CAD build for the part. Positions are in the model's coordinates, mm. Face numbers are marked on the shaded views. A direction names the side the tool comes from. Round coordinates to 2 decimals unless told otherwise and drop trailing zeros. Order: outer loops, then holes, each group sorted by start corner. A loop starts at its lowest first (then second) coordinate and runs counter-clockwise, first axis right, second up. Notation, with made-up numbers: (65, -25.75) -> (76, -25.75) arc R13 cw to (76, -9.75) -> close; hole circle Ø4 at (77, 28). An arc over 180 degrees is marked (long way). Return JSON: item names as keys, results as strings. Group by question number.
Q1. Cut at C-C (z = -7.5). Write the cut outline in (x, y), then the cut area to 3 significant figures.
Q2. Cut at B-B (y = 0.35). Write the cut outline in (x, z), then the cut area to 3 significant figures.
Q3. Cut at D-D (x = 6.5). Write the cut outline in (y, z), then the cut area to 3 significant figures.
Q4. Mould opens along X. For the marked faces 3, 4, 5 and 6 say: +X half, -X half, draft (parallel to the pull), parting line (faces both ways), or undercut.
Q5. Which spindle directions (+Z, -Z, +X, -X, +Y, -Y) get a long thin tool onto all of the face, cutting with end or side? Do the marked faces 1 and 2. Say none if no direction does.
Q6. Cut at A-A (x = 5). Write the cut outline in (y, z), then the cut area to 3 significant figures.
Q7. Probe line 1 along X through (y, z) = (-0.2, -7.5); line 2 along X through (y, z) = (0.95, -7.5); line 3 along Z through (x, y) = (5, 0.7). List the from-to ranges inside material, lowest first.
from build123d import *

# Parameters (mm, degrees)
SKETCH1_W             = 10
SKETCH1_H             = 15
BOSS_EXTRUDE1_DEPTH   = 1.6
FILLET1_R             = 1.5
SKETCH2_R             = 3.45
BOSS_EXTRUDE2_DEPTH   = 1.4
M3X0_5_TAPPED_HOLE1_D = 2.5


with BuildPart() as part:
    # Sketch1 → Boss-Extrude1 (new body)
    with BuildSketch(Plane(origin=(0, 0, 0), x_dir=(1, 0, 0), z_dir=(0, 1, 0))):
        with Locations((5, 7.5)):
            Rectangle(SKETCH1_W, SKETCH1_H)
    extrude(amount=BOSS_EXTRUDE1_DEPTH)

    # Fillet1
    fillet1_edges = [part.edges().sort_by_distance(p)[0] for p in [
        (0, 0.8, -15),
        (10, 0.8, -15),
        (10, 0.8, 0),
        (0, 0.8, 0),
    ]]
    fillet(fillet1_edges, radius=FILLET1_R)

    # Sketch2 → Boss-Extrude2 (add)
    with BuildSketch(Plane.XZ):
        with Locations(Location((5, -7.5, 0), (0, 0, 270))):
            Circle(SKETCH2_R)
    extrude(amount=BOSS_EXTRUDE2_DEPTH)

    # M3x0.5 Tapped Hole1 (through all)
    with Locations(Plane(origin=(0, 1.6, 0), x_dir=(1, 0, 0), z_dir=(0, 1, 0))):
        with Locations((5, 7.5)):
            Hole(M3X0_5_TAPPED_HOLE1_D / 2)


solid = part.part
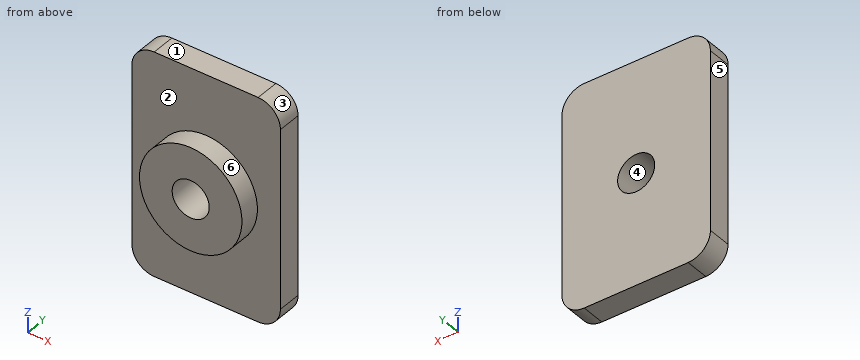
Solution:
{
 "1": {"outline": "(0, 0) -> (1.55, 0) -> (1.55, -1.4) -> (3.75, -1.4) -> (3.75, 1.6) -> (0, 1.6) -> close; (6.25, -1.4) -> (8.45, -1.4) -> (8.45, 0) -> (10, 0) -> (10, 1.6) -> (6.25, 1.6) -> close", "area": "18.2 mm²"},
 "2": {"outline": "(0, -13.5) arc R1.5 ccw to (1.5, -15) -> (8.5, -15) arc R1.5 ccw to (10, -13.5) -> (10, -1.5) arc R1.5 ccw to (8.5, 0) -> (1.5, 0) arc R1.5 ccw to (0, -1.5) -> close; hole circle Ø2.5 at (5, -7.5)", "area": "143 mm²"},
 "3": {"outline": "(-1.4, -10.61) -> (0, -10.61) -> (0, -15) -> (1.6, -15) -> (1.6, 0) -> (0, 0) -> (0, -4.39) -> (-1.4, -4.39) -> close", "area": "32.7 mm²"},
 "4": {"face 3": "+X half", "face 4": "undercut", "face 5": "-X half", "face 6": "parting line"},
 "5": {"face 1": "+Z, +X, -X, +Y, -Y", "face 2": "-Y"},
 "6": {"outline": "(-1.4, -10.95) -> (0, -10.95) -> (0, -15) -> (1.6, -15) -> (1.6, -8.75) -> (-1.4, -8.75) -> close; (-1.4, -6.25) -> (1.6, -6.25) -> (1.6, 0) -> (0, 0) -> (0, -4.05) -> (-1.4, -4.05) -> close", "area": "26.2 mm²"},
 "7": {"line 1": "x = 1.55 to 3.75, 6.25 to 8.45", "line 2": "x = 0 to 3.75, 6.25 to 10", "line 3": "z = -15 to -8.75, -6.25 to 0"}
}
